Drawing for the job (mm, zero at the part's lowest x, y, z). A direction names the side the tool comes from. Give positions to 0.01 mm unless a question says otherwise; leave off trailing zeros. Loops run counter-clockwise (first coordinate to the right, second up) from the corner with the lowest first, then second, coordinate; pieces in that order, holes last.
1) Flat gauge pins, fed straight in: P1, Ø0.8, axis at y = 2, z = 0.5, coming from the +X side; P2, Ø1.5, axis at x = 11, y = 1, coming from the -Z side; P3, Ø0.5, axis at y = 1, z = 6.5, coming from the -X side. Where does each tip first touch, or does it go through?
2) Band-saw the part on C-C on y = 1.6. List the corners of the cut face in (x, z), then the cut area to 3 significant figures.
3) Band-saw the part on D-D on x = 11.5. List the corners of the cut face in (y, z), then the cut area to 3 significant figures.
4) Band-saw the part on A-A on x = 7.5. List the corners of the cut face in (y, z), then the cut area to 3 significant figures.
5) Band-saw the part on B-B on z = 6.25. List the corners of the cut face in (x, y), then the cut area to 3 significant figures.
6) Wall check: line 1 (X direction, y = 2.25, z = 5); line 2 (X direction, y = 1.75, z = 6.25); line 3 (Z direction, x = 6.25, y = 2.45). Give the ranges that are in metal, low to high.
7) Two-plate mould, pull along X, no slides. Class the marked faces 1, 2 and 3: +X half, -X half, draft (parallel to the pull), parting line (faces both ways), or undercut.
8) 3-axis set-ups, long thin cutter, end or side, ignore diameter. For the marked faces 4, 5 and 6: which of +Z, -Z, +X, -X, +Y, -Y reach the whole face in a straight line?
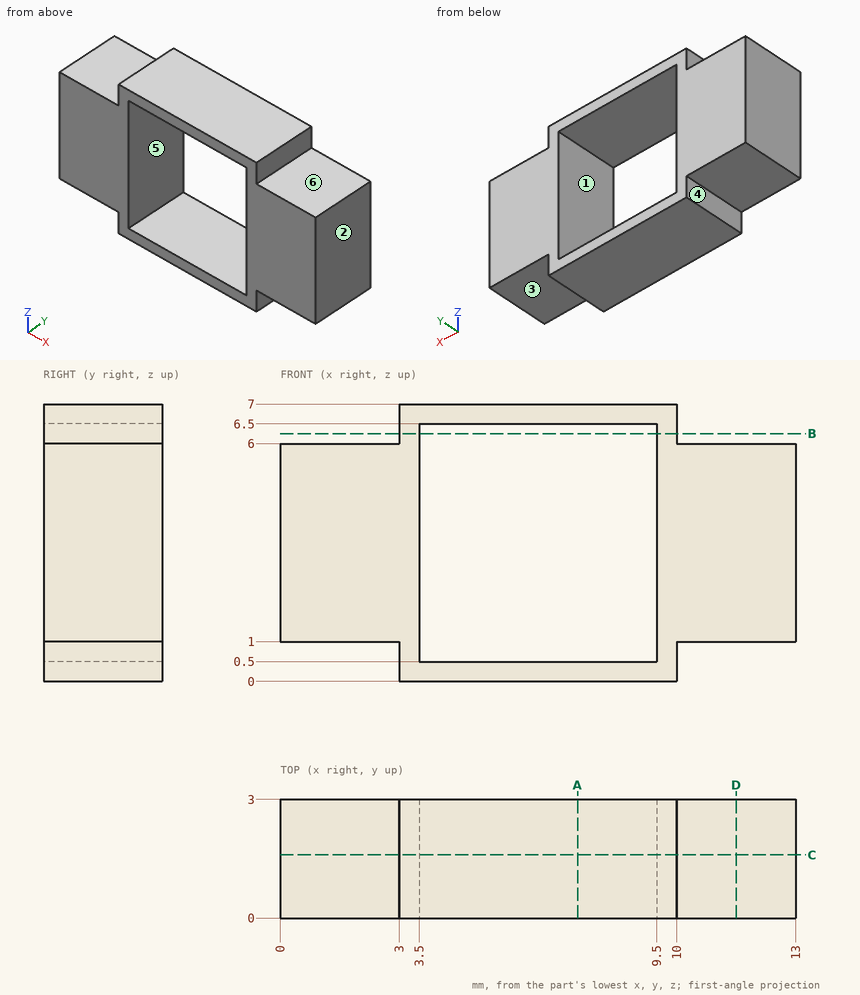
Findings below:
1. P1: stops at x = 10
1. P2: stops at z = 1
1. P3: stops at x = 3
2. outline: (0, 1) - (3, 1) - (3, 0) - (10, 0) - (10, 1) - (13, 1) - (13, 6) - (10, 6) - (10, 7) - (3, 7) - (3, 6) - (0, 6) - close; hole (3.5, 0.5) - (9.5, 0.5) - (9.5, 6.5) - (3.5, 6.5) - close
2. area: 43.0 mm2
3. outline: (0, 1) - (3, 1) - (3, 6) - (0, 6) - close
3. area: 15.0 mm2
4. outline: (0, 0) - (3, 0) - (3, 0.5) - (0, 0.5) - close; (0, 6.5) - (3, 6.5) - (3, 7) - (0, 7) - close
4. area: 3.00 mm2
5. outline: (3, 0) - (3.5, 0) - (3.5, 3) - (3, 3) - close; (9.5, 0) - (10, 0) - (10, 3) - (9.5, 3) - close
5. area: 3.00 mm2
6. line 1: x = 0 to 3.5, 9.5 to 13
6. line 2: x = 3 to 3.5, 9.5 to 10
6. line 3: z = 0 to 0.5, 6.5 to 7
7. face 1: undercut
7. face 2: +X half
7. face 3: draft
8. face 4: -Z, -X, +Y, -Y
8. face 5: +Y, -Y
8. face 6: +Z, +X, +Y, -Y
